Part model, mm, in its own coordinate system. A direction names the side the tool comes from. Round coordinates to 2 decimals unless told otherwise and drop trailing zeros. Loops run counter-clockwise (first coordinate to the right, second up) from the corner with the lowest first, then second, coordinate; pieces in that order, holes last. Notation, with made-up numbers: (72, 71.25) - (85, 71.25) arc R27 cw to (85, 101.25) - close; hole circle Ø11 at (20, 61.5). An arc over 180 degrees is marked (long way). Write each question's results on one line, items separated by ' | '. Start each with the question number.
(1) Flat gauge pins, fed straight in: P1, Ø1.5, axis at x = 5.5, y = 19, coming from the -Z side; P2, Ø1.5, axis at x = 19, y = 29.5, coming from the -Z side; P3, Ø2, axis at x = 17.5, z = 1, coming from the -Y side; P4, Ø1, axis at y = 16.5, z = -81, coming from the -X side. Where does each tip first touch, or does it go through?
(2) Tool access for faces 1 (the face through (22, 24, 0)), 2 (the face through (18, 10, 1)), 3 (the face through (18, 38, -81)), 4 (the face through (30, 31, -79)): list every direction of +Z, -Z, +X, -X, +Y, -Y with a clear straight run to the whole face (end or side of a thin tool).
(3) Cut at D-D, the plane z = -3. List the corners of the cut face in (x, y), then the cut area to 3 significant figures.
(4) Drill centre lines: L1, parallel to X at y = 30.5, z = -42; L2, parallel to Z at x = 28.5, y = 23.5; L3, parallel to Z at x = 1, y = 16.5. Where is each one in solid material? Low to high.
(5) Cut at B-B, the plane x = 12. List the corners of the cut face in (y, z), then the cut area to 3 significant figures.
(6) Mould opens along Y. For faces 5 (the face through (18, 2, -81)), 6 (the face through (14, 28, 1)), 7 (the face through (38, 20, -38)), 8 (the face through (8, 15, 1)) say: released by +Y, released by -Y, zero draft, split by the parting line, or undercut.
(7) Cut at C-C, the plane x = 16.5. List the corners of the cut face in (y, z).
(8) Cut at A-A, the plane y = 32. List the corners of the cut face in (x, z).
from build123d import *

# Parameters (mm, degrees)
SKETCH1_W           = 40
SKETCH1_H           = 82
SKETCH1_W_2         = 36
SKETCH1_H_2         = 78
BOSS_EXTRUDE1_DEPTH = 40
SKETCH2_W           = 20
SKETCH2_H           = 10
SKETCH2_W_2         = 14
SKETCH2_H_2         = 12
CUT_EXTRUDE1_DEPTH  = 20
SKETCH4_W           = 36
SKETCH4_H           = 36
SKETCH4_W_2         = 32
SKETCH4_H_2         = 32
BOSS_EXTRUDE2_DEPTH = 2
SKETCH3_W           = 24
SKETCH3_H           = 6
CUT_EXTRUDE2_DEPTH  = 2


with BuildPart() as part:
    # Sketch1 → Boss-Extrude1 (new body)
    with BuildSketch(Plane(origin=(0, 0, 0), x_dir=(1, 0, 0), z_dir=(0, 1, 0))):
        with Locations((18, 39)):
            Rectangle(SKETCH1_W, SKETCH1_H)
        with Locations((18, 39)):
            Rectangle(SKETCH1_W_2, SKETCH1_H_2, mode=Mode.SUBTRACT)
    extrude(amount=BOSS_EXTRUDE1_DEPTH)

    # Sketch2 → Cut-Extrude1 (cut)
    with BuildSketch(Plane.XY.offset(2)):
        with Locations((18, 15)):
            Rectangle(SKETCH2_W, SKETCH2_H)
        with Locations((7, 28)):
            Rectangle(SKETCH2_W_2, SKETCH2_H_2)
    extrude(amount=-CUT_EXTRUDE1_DEPTH, mode=Mode.SUBTRACT)

    # Sketch4 → Boss-Extrude2 (add)
    with BuildSketch(Plane(origin=(0, 0, -80), x_dir=(-1, 0, 0), z_dir=(0, 0, -1))):
        with Locations((-18, 20)):
            Rectangle(SKETCH4_W, SKETCH4_H)
        with Locations((-18, 20)):
            Rectangle(SKETCH4_W_2, SKETCH4_H_2, mode=Mode.SUBTRACT)
    extrude(amount=BOSS_EXTRUDE2_DEPTH)

    # Sketch3 → Cut-Extrude2 (cut)
    with BuildSketch(Plane(origin=(0, 0, -80), x_dir=(-1, 0, 0), z_dir=(0, 0, -1))):
        with Locations((-18, 31)):
            Rectangle(SKETCH3_W, SKETCH3_H)
    extrude(amount=-CUT_EXTRUDE2_DEPTH, mode=Mode.SUBTRACT)


solid = part.part
A:
1) P1: z = -80 | P2: z = 0 | P3: y = 0 | P4: x = 0
2) face 1: +Y, -Y | face 2: +Z | face 3: -Z, +X, -X, +Y | face 4: -Z
3) outline: (-2, 0) - (0, 0) - (0, 40) - (-2, 40) - close; (36, 0) - (38, 0) - (38, 40) - (36, 40) - close | area: 160 mm2
4) L1: -2 to 0, 36 to 38 | L2: -80 to -78, 0 to 2 | L3: -82 to -78, 0 to 2
5) outline: (0, -80) - (2, -80) - (2, -82) - (4, -82) - (4, -80) - (28, -80) - (28, -78) - (0, -78) - close; (0, 0) - (10, 0) - (10, 2) - (0, 2) - close; (20, 0) - (22, 0) - (22, 2) - (20, 2) - close; (34, -80) - (36, -80) - (36, -82) - (38, -82) - (38, -80) - (40, -80) - (40, -78) - (34, -78) - close; (34, 0) - (40, 0) - (40, 2) - (34, 2) - close | area: 112 mm2
6) face 5: released by -Y | face 6: undercut | face 7: zero draft | face 8: undercut
7) outline: (0, -80) - (2, -80) - (2, -82) - (4, -82) - (4, -80) - (28, -80) - (28, -78) - (0, -78) - close; (0, 0) - (10, 0) - (10, 2) - (0, 2) - close; (20, 0) - (40, 0) - (40, 2) - (20, 2) - close; (34, -80) - (36, -80) - (36, -82) - (38, -82) - (38, -80) - (40, -80) - (40, -78) - (34, -78) - close
8) outline: (-2, -80) - (0, -80) - (0, -82) - (2, -82) - (2, -80) - (6, -80) - (6, -78) - (0, -78) - (0, 2) - (-2, 2) - close; (14, 0) - (36, 0) - (36, -78) - (30, -78) - (30, -80) - (34, -80) - (34, -82) - (36, -82) - (36, -80) - (38, -80) - (38, 2) - (14, 2) - close
